from build123d import *

# Parameters (mm, degrees)
F0_W      = 130
F0_H      = 78
F14_DEPTH = 150
F1_SIZE   = 5
F2_DEPTH  = 67.5
F4_R      = 6
F5_DEPTH  = 150.001
F6_R      = 7
F6_R_2    = 3
F7_DEPTH  = 25
F9_R      = 2.5
F10_DEPTH = 10.501
F11_DEPTH = 25
F11_TAPER = -27
F12_R     = 3
F13_DEPTH = 25


with BuildPart() as f14:
    # F0 (on Top) → F14 (new body)
    with BuildSketch(Plane.XY):
        Rectangle(F0_W, F0_H)
    extrude(amount=-F14_DEPTH)

    # F1
    f1_edges = [f14.edges().sort_by_distance(p)[0] for p in [
        (65, 0, 0),
        (-65, 0, 0),
        (0, 39, 0),
    ]]
    chamfer(f1_edges, length=F1_SIZE)

    # F15 (on face) → F2 (cut)
    with BuildSketch(Plane(origin=(0, 39, 0), x_dir=(-1, 0, 0), z_dir=(0, 1, 0))):
        Polygon((-16, -9), (-56, -9), (-56, -150), (56, -150), (56, -9), (16, -9), (16, -22), (-16, -22), align=None)
    extrude(amount=-F2_DEPTH, mode=Mode.SUBTRACT)

    # F4 (on face) → F5 (cut, through all)
    with BuildSketch(Plane.XY):
        with Locations((5.5, 6.5)):
            Circle(F4_R)
    extrude(amount=-F5_DEPTH, mode=Mode.SUBTRACT)

    # F6 (on face) → F7 (cut)
    with BuildSketch(Plane.XY):
        with Locations((5.5, 6.5)):
            Circle(F6_R)
        with Locations((-29.3, -28.3)):
            Circle(F6_R_2)
        with Locations((-29.3, 41.3)):
            Circle(F6_R_2)
        with Locations((40.3, 41.3)):
            Circle(F6_R_2)
        with Locations((40.3, -28.3)):
            Circle(F6_R_2)
    extrude(amount=-F7_DEPTH, mode=Mode.SUBTRACT)

    # F9 (on face) → F10 (cut, through all)
    with BuildSketch(Plane(origin=(0, -28.5, 0), x_dir=(-1, 0, 0), z_dir=(0, 1, 0))):
        with Locations((-28.5, -94)):
            Circle(F9_R)
        with Locations((-28.5, -107)):
            Circle(F9_R)
        with Locations((17.5, -94)):
            Circle(F9_R)
        with Locations((17.5, -107)):
            Circle(F9_R)
    extrude(amount=-F10_DEPTH, mode=Mode.SUBTRACT)

    # F16 (on face) → F11 (cut)
    with BuildSketch(Plane.XZ.offset(39)):
        with BuildLine():
            Line((17.5, -107), (-5, -107))
            ThreePointArc((-5, -107), (-12.0710678119, -109.9289321881), (-15, -117))
            Line((-15, -117), (-15, -150))
            Line((-15, -150), (27.5, -150))
            Line((27.5, -150), (27.5, -117))
            ThreePointArc((27.5, -117), (24.5710678119, -109.9289321881), (17.5, -107))
        make_face()
    extrude(amount=-F11_DEPTH, taper=F11_TAPER, mode=Mode.SUBTRACT)

    # F12 (on face) → F13 (cut)
    with BuildSketch(Plane.XY):
        with Locations((-29.3, 24)):
            Circle(F12_R)
        with Locations((40.3, 24)):
            Circle(F12_R)
    extrude(amount=-F13_DEPTH, mode=Mode.SUBTRACT)


solid = f14.part
Verification items for the finished model (mm, model axes). A direction names the side the tool comes from. Give positions to 0.01 mm unless a question says otherwise; leave off trailing zeros. Loops run counter-clockwise (first coordinate to the right, second up) from the corner with the lowest first, then second, coordinate; pieces in that order, holes last.
1) Sectioned sample at A-A, the plane z = -94. Enter the section's corners in (x, y).
2) Sectioned sample at D-D, the plane y = -4. Enter the section's corners in (x, z).
3) Set-up check for faces 5 (the flat face through (-4, 6, -22)), 6 (the cylindrical face through (-27.916, -30.962, -9.547)), 7 (the flat face through (-58, 39, -72)): record each of +Z, -Z, +X, -X, +Y, -Y from which the full face is reachable in a straight line by a thin tool's end or side.
4) Thickness scan on line 1 along Y through (x, z) = (40.3, -5.5); line 2 along X through (y, z) = (12.5, -77); line 3 along Y through (x, z) = (-29, -2). Record the ranges inside material, lowest first.
5) Sectioned sample at B-B, the plane x = -29.3. Enter the section's corners in (y, z).
6) Sectioned sample at C-C, the plane y = 6.5. Enter the section's corners in (x, z).
7) Draft check along Z on faces 1 (the cylindrical face through (-17.17, -33.68, -91.52)), 2 (the cylindrical face through (-19, -34, -105)), 3 (the conical face through (26.162, -34.843, -108.526)), 4 (the flat face through (16, 6, -16)). Enter one of: pulls with the +Z half, pulls with the -Z half, needs draft (parallel to the pull), parting line crosses it, or undercut.
8) Depth check by flat-ended pin: pin 1 Ø10 at (x, y) = (-29.5, 8.5) entering from -Z; pin 2 Ø0.8 at (x, y) = (40.5, -30) entering from +Z; pin 3 Ø6.5 at (x, z) = (-17.5, -94) entering from +Y; pin 4 Ø6 at (x, z) = (-17.5, -107) entering from -Y. Enter the tip coordinate at first touch or a pass-through.
Answers:
1. outline: (-65, -39) - (-20, -39) - (-20, -28.5) - (-56, -28.5) - (-56, 39) - (-65, 39) - close; (-15, -39) - (26, -39) - (26, -28.5) - (-15, -28.5) - close; (31, -39) - (65, -39) - (65, 39) - (56, 39) - (56, -28.5) - (31, -28.5) - close
2. outline: (-65, -150) - (-56, -150) - (-56, -9) - (-16, -9) - (-16, -22) - (16, -22) - (16, -9) - (56, -9) - (56, -150) - (65, -150) - (65, -5) - (60, 0) - (-60, 0) - (-65, -5) - close
3. face 5: -Z, +Y
3. face 6: +Z
3. face 7: +Z, -Z, +X, -X, +Y
4. line 1: y = -39 to -31.3, -25.3 to 21, 27 to 38.3
4. line 2: x = -65 to -56, 56 to 65
4. line 3: y = -39 to -31.28, -25.32 to 21.02, 26.98 to 36
5. outline: (-39, -150) - (-28.5, -150) - (-28.5, -25) - (-31.3, -25) - (-31.3, 0) - (-39, 0) - close; (-25.3, -9) - (21, -9) - (21, 0) - (-25.3, 0) - close; (27, -9) - (38.3, -9) - (38.3, -4.3) - (34, 0) - (27, 0) - close
6. outline: (-65, -150) - (-56, -150) - (-56, -9) - (-16, -9) - (-16, -22) - (-1.5, -22) - (-1.5, 0) - (-60, 0) - (-65, -5) - close; (12.5, -22) - (16, -22) - (16, -9) - (56, -9) - (56, -150) - (65, -150) - (65, -5) - (60, 0) - (12.5, 0) - close
7. face 1: undercut
7. face 2: undercut
7. face 3: pulls with the -Z half
7. face 4: needs draft
8. pin 1: stops at z = -9
8. pin 2: stops at z = -25
8. pin 3: stops at y = -28.5
8. pin 4: stops at y = -39
